Can you work these out from the model? Positions are in its coordinate system, mm. Face numbers are marked on the shaded views. A direction names the side the tool comes from. Coordinates: 2 decimals unless noted, no trailing zeros. Order: outer loops, then holes, each group sorted by start corner. A loop starts at its lowest first (then second) coordinate and runs counter-clockwise, first axis right, second up. Notation, with made-up numbers: (2, 12) - (38, 12) arc R24 cw to (38, 36) - close; hole circle Ø8 at (4.25, 72.25). An arc over 180 degrees is marked (long way). Return JSON: item names as keys, results as strings. Group by question number.
1) Which directions (+Z, -Z, +X, -X, +Y, -Y) give clear straight access to the entire face, cutting with the end or side of a thin tool? Please do the marked faces 4, 5, 6, 7 and 8.
2) If we mould it in two halves opening along X, with no side actions, what happens to the marked faces 1, 2 and 3? For each: pulls with the +X half, pulls with the -X half, needs draft (parallel to the pull), parting line crosses it, or undercut.
3) Imagine slicing it at A-A (x = 12.5). Write out the boundary of the cut face in (y, z).
4) Imagine slicing it at C-C (x = 18.5). Write out the boundary of the cut face in (y, z).
5) For pin 1 Ø2 at (y, z) = (-3.5, -5) entering from +X; pin 2 Ø4.5 at (x, y) = (1, 1.5) entering from -Z; pin 3 Ø10 at (x, z) = (2, -2) entering from -Y, each with a flat end and sliding along its axis, tell me the tip position at first contact or that it passes through.
6) Imagine slicing it at D-D (z = 0). Give the number of separate pieces and of enclosed holes in the cut face, and give its area (3 significant figures).
7) If I drill on line 1 along Z through (x, y) = (0, -12.25); line 2 along Z through (x, y) = (0, 21), over which ranges is the centre line in solid material (lowest first)?
8) Imagine slicing it at B-B (z = -18). Write out the boundary of the cut face in (x, y), and give its area (3 significant figures).
```python
from build123d import *

# Parameters (mm, degrees)
BOSS_EXTRUDE1_DEPTH         = 22.86
BOSS_EXTRUDE1_DEPTH_BACK    = 22.86
SKETCH1_W                   = 45.72
SKETCH1_H                   = 45.72
SKETCH4_R                   = 20.287199642
CUT_EXTRUDE1_DEPTH          = 7.62
SKETCH5_R                   = 10.041617815
CUT_EXTRUDE2_DEPTH          = 15.24
CIRPATTERN1_COUNT           = 4
CIRPATTERN2_COUNT           = 2
CIRPATTERN2_ANGLE           = 90
CIRPATTERN2_COPY_1_SKETCH_R = 20.287199642
CIRPATTERN2_COPY_1_DEPTH    = 7.62
CIRPATTERN2_COPY_2_SKETCH_R = 20.287199642
CIRPATTERN2_COPY_2_DEPTH    = 7.62
CIRPATTERN2_COPY_3_SKETCH_R = 20.287199642
CIRPATTERN2_COPY_3_DEPTH    = 7.62
CIRPATTERN2_COPY_4_SKETCH_R = 10.041617815
CIRPATTERN2_COPY_4_DEPTH    = 15.24
CIRPATTERN2_COPY_5_SKETCH_R = 10.041617815
CIRPATTERN2_COPY_5_DEPTH    = 15.24
CIRPATTERN2_COPY_6_SKETCH_R = 10.041617815
CIRPATTERN2_COPY_6_DEPTH    = 15.24


with BuildPart() as part:
    # Sketch1 → Boss-Extrude1 (new, two sides: drawn at the far end of the back side and taken through both)
    with BuildSketch(Plane.XY.offset(-BOSS_EXTRUDE1_DEPTH_BACK)):
        Rectangle(SKETCH1_W, SKETCH1_H)
    extrude(amount=BOSS_EXTRUDE1_DEPTH + BOSS_EXTRUDE1_DEPTH_BACK)

    # Sketch4 → Cut-Extrude1 (cut)
    with BuildSketch(Plane.XY.offset(22.86)):
        Circle(SKETCH4_R)
    cut_extrude1 = extrude(amount=-CUT_EXTRUDE1_DEPTH, mode=Mode.SUBTRACT)

    # Sketch5 → Cut-Extrude2 (cut)
    with BuildSketch(Plane.XY.offset(22.86)):
        Circle(SKETCH5_R)
    cut_extrude2 = extrude(amount=-CUT_EXTRUDE2_DEPTH, mode=Mode.SUBTRACT)

    # CirPattern1: Cut-Extrude1, Cut-Extrude2 ×4 about axis
    cirpattern1_axis = Axis((0, 0, 0), (0, 1, 0))
    add([cut_extrude1.rotate(cirpattern1_axis, i * 360 / CIRPATTERN1_COUNT) for i in range(1, CIRPATTERN1_COUNT)], mode=Mode.SUBTRACT)
    add([cut_extrude2.rotate(cirpattern1_axis, i * 360 / CIRPATTERN1_COUNT) for i in range(1, CIRPATTERN1_COUNT)], mode=Mode.SUBTRACT)

    # CirPattern2: Cut-Extrude1, Cut-Extrude2 ×2 about axis
    cirpattern2_axis = Axis((-25.146, 0, 0), (1, 0, 0))
    add([cut_extrude1.rotate(cirpattern2_axis, i * CIRPATTERN2_ANGLE / (CIRPATTERN2_COUNT - 1)) for i in range(1, CIRPATTERN2_COUNT)], mode=Mode.SUBTRACT)
    add([cut_extrude2.rotate(cirpattern2_axis, i * CIRPATTERN2_ANGLE / (CIRPATTERN2_COUNT - 1)) for i in range(1, CIRPATTERN2_COUNT)], mode=Mode.SUBTRACT)

    # CirPattern2 copy 1 sketch → CirPattern2 copy 1 (cut)
    with BuildSketch(Plane.YZ.offset(22.86)):
        Circle(CIRPATTERN2_COPY_1_SKETCH_R)
    extrude(amount=-CIRPATTERN2_COPY_1_DEPTH, mode=Mode.SUBTRACT)

    # CirPattern2 copy 2 sketch → CirPattern2 copy 2 (cut)
    with BuildSketch(Plane(origin=(0, 22.86, 0), x_dir=(-1, 0, 0), z_dir=(0, 1, 0))):
        Circle(CIRPATTERN2_COPY_2_SKETCH_R)
    extrude(amount=-CIRPATTERN2_COPY_2_DEPTH, mode=Mode.SUBTRACT)

    # CirPattern2 copy 3 sketch → CirPattern2 copy 3 (cut)
    with BuildSketch(Plane(origin=(-22.86, 0, 0), x_dir=(0, -1, 0), z_dir=(-1, 0, 0))):
        Circle(CIRPATTERN2_COPY_3_SKETCH_R)
    extrude(amount=-CIRPATTERN2_COPY_3_DEPTH, mode=Mode.SUBTRACT)

    # CirPattern2 copy 4 sketch → CirPattern2 copy 4 (cut)
    with BuildSketch(Plane.YZ.offset(22.86)):
        Circle(CIRPATTERN2_COPY_4_SKETCH_R)
    extrude(amount=-CIRPATTERN2_COPY_4_DEPTH, mode=Mode.SUBTRACT)

    # CirPattern2 copy 5 sketch → CirPattern2 copy 5 (cut)
    with BuildSketch(Plane(origin=(0, 22.86, 0), x_dir=(-1, 0, 0), z_dir=(0, 1, 0))):
        Circle(CIRPATTERN2_COPY_5_SKETCH_R)
    extrude(amount=-CIRPATTERN2_COPY_5_DEPTH, mode=Mode.SUBTRACT)

    # CirPattern2 copy 6 sketch → CirPattern2 copy 6 (cut)
    with BuildSketch(Plane(origin=(-22.86, 0, 0), x_dir=(0, -1, 0), z_dir=(-1, 0, 0))):
        Circle(CIRPATTERN2_COPY_6_SKETCH_R)
    extrude(amount=-CIRPATTERN2_COPY_6_DEPTH, mode=Mode.SUBTRACT)


solid = part.part
```
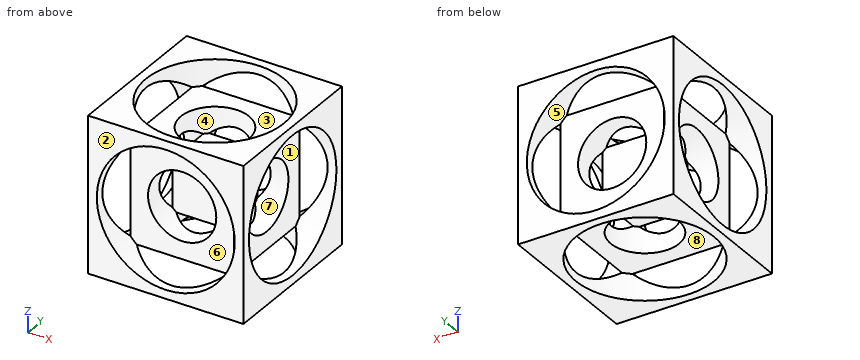
Calculated:
{
 "1": {"face 4": "+Z", "face 5": "+Y", "face 6": "-Y", "face 7": "+X", "face 8": "-Z"},
 "2": {"face 1": "pulls with the +X half", "face 2": "needs draft", "face 3": "undercut"},
 "3": {"outline": "(-22.86, -22.86) - (-15.98, -22.86) - (-15.98, -15.98) - (-22.86, -15.98) - close; (-22.86, 15.98) - (-15.98, 15.98) - (-15.98, 22.86) - (-22.86, 22.86) - close; (-15.24, -15.24) - (15.24, -15.24) - (15.24, 15.24) - (-15.24, 15.24) - close; (15.98, -22.86) - (22.86, -22.86) - (22.86, -15.98) - (15.98, -15.98) - close; (15.98, 15.98) - (22.86, 15.98) - (22.86, 22.86) - (15.98, 22.86) - close; hole circle Ø20.08 at (0, 0)"},
 "4": {"outline": "(-22.86, -22.86) - (-8.33, -22.86) - (-8.33, -18.5) arc R20.29 cw to (-18.5, -8.33) - (-22.86, -8.33) - close; (-22.86, 8.33) - (-18.5, 8.33) arc R20.29 cw to (-8.33, 18.5) - (-8.33, 22.86) - (-22.86, 22.86) - close; (8.33, -22.86) - (22.86, -22.86) - (22.86, -8.33) - (18.5, -8.33) arc R20.29 cw to (8.33, -18.5) - close; (8.33, 18.5) arc R20.29 cw to (18.5, 8.33) - (22.86, 8.33) - (22.86, 22.86) - (8.33, 22.86) - close"},
 "5": {"pin 1": "x = 7.62", "pin 2": "z = -7.62", "pin 3": "y = -7.62"},
 "6": {"separate pieces": "9", "enclosed holes": "0", "area": "367 mm2"},
 "7": {"line 1": "-15.24 to -10.04, 10.04 to 15.24", "line 2": "-22.86 to -20.29, 20.29 to 22.86"},
 "8": {"outline": "(-22.86, -22.86) - (-9.36, -22.86) - (-9.36, -18) arc R20.29 cw to (-18, -9.36) - (-22.86, -9.36) - close; (-22.86, 9.36) - (-18, 9.36) arc R20.29 cw to (-9.36, 18) - (-9.36, 22.86) - (-22.86, 22.86) - close; (9.36, -22.86) - (22.86, -22.86) - (22.86, -9.36) - (18, -9.36) arc R20.29 cw to (9.36, -18) - close; (9.36, 18) arc R20.29 cw to (18, 9.36) - (22.86, 9.36) - (22.86, 22.86) - (9.36, 22.86) - close", "area": "549 mm2"}
}
